The listing builds one solid part. Answer for the finished solid, in the listing's coordinates (mm). A direction names the side the tool comes from. Give positions to 0.01 mm unless a question says otherwise; leave off trailing zeros. Write each loop counter-clockwise with the first axis right and the second up, starting at its lowest first coordinate (ties: lowest second). Pieces come first, ordered by that corner, then holes. Notation, with made-up numbers: M -36.75,66 L 6.25,66 A33 ccw 6.25,105 Z; hole C -5.5,47 d5. An arc over 180 degrees is marked long. Return JSON: item names as keys, results as strings.
from build123d import *

# Parameters (mm, degrees)
SKETCH1_W           = 50.8
SKETCH1_H           = 50.8
SKETCH1_W_2         = 44.45
SKETCH1_H_2         = 44.45
BOSS_EXTRUDE1_DEPTH = 279.4
SKETCH2_R           = 6.35
SKETCH2_R_2         = 12.7
CUT_EXTRUDE1_DEPTH  = 289.488543967
CHAMFER1_SIZE       = 25.4
SKETCH3_R           = 3.175
CUT_EXTRUDE2_DEPTH  = 289.488543967
SKETCH4_W           = 25.4
SKETCH4_H           = 55.88
CUT_EXTRUDE3_DEPTH  = 289.488543967
CHAMFER2_SIZE       = 12.7
CUT_EXTRUDE5_REACH  = 290.489
SKETCH6_R           = 2.5796875


with BuildPart() as part:
    # Sketch1 → Boss-Extrude1 (new body)
    with BuildSketch(Plane(origin=(0, 0, 0), x_dir=(1, 0, 0), z_dir=(0, 1, 0))):
        with Locations((25.4, 25.4)):
            Rectangle(SKETCH1_W, SKETCH1_H)
        with Locations((25.4, 25.4)):
            Rectangle(SKETCH1_W_2, SKETCH1_H_2, mode=Mode.SUBTRACT)
    extrude(amount=BOSS_EXTRUDE1_DEPTH)

    # Sketch2 → Cut-Extrude1 (cut, through all)
    with BuildSketch(Plane(origin=(0, 0, -50.8), x_dir=(-1, 0, 0), z_dir=(0, 0, -1))):
        with Locations((-12.7, 25.4)):
            Circle(SKETCH2_R)
        with Locations((-25.4, 254)):
            Circle(SKETCH2_R_2)
    extrude(amount=-CUT_EXTRUDE1_DEPTH, mode=Mode.SUBTRACT)

    # Chamfer1
    # the kernel refuses this chamfer: 25.4 mm, written as the material it takes off along each edge
    with BuildSketch(Plane(origin=(50.8, 0, 65.320747894), x_dir=(-0.9996219169112966, -0.02749587661058637, 0), z_dir=(0, 0, -1))) as chamfer1_piece_1:
        Polygon((CHAMFER1_SIZE * 0.999621916911, CHAMFER1_SIZE * 0.0274958766106), (-CHAMFER1_SIZE * 0.0274958766106, CHAMFER1_SIZE * 0.999621916911), (0, 0), align=None)
    extrude(amount=181.441495789, mode=Mode.SUBTRACT)

    # Sketch3 → Cut-Extrude2 (cut, through all)
    with BuildSketch(Plane(origin=(0, 0, -50.8), x_dir=(-1, 0, 0), z_dir=(0, 0, -1))):
        with Locations((-38.1, 101.6)):
            Circle(SKETCH3_R)
    extrude(amount=-CUT_EXTRUDE2_DEPTH, mode=Mode.SUBTRACT)

    # Sketch4 → Cut-Extrude3 (cut, through all)
    with BuildSketch(Plane.ZY):
        with Locations((-38.1, 251.46)):
            Rectangle(SKETCH4_W, SKETCH4_H)
    extrude(amount=-CUT_EXTRUDE3_DEPTH, mode=Mode.SUBTRACT)

    # Chamfer2
    chamfer2_edges = [part.edges().sort_by_distance(p)[0] for p in [
        (49.2125, 279.4, -25.4),
        (1.5875, 279.4, -25.4),
    ]]
    chamfer(chamfer2_edges, length=CHAMFER2_SIZE)

    # Sketch6 → Cut-Extrude5 (cut, up to next)
    with BuildSketch(Plane.XY, mode=Mode.PRIVATE) as cut_extrude5_sk1:
        with Locations((7.439487758, 271.960512242)):
            Circle(SKETCH6_R)
    cut_extrude5_tool1 = extrude(cut_extrude5_sk1.sketch, amount=-CUT_EXTRUDE5_REACH, mode=Mode.PRIVATE) & part.part
    # Sketch6 → Cut-Extrude5 (cut, up to next)
    with BuildSketch(Plane.XY, mode=Mode.PRIVATE) as cut_extrude5_sk2:
        with Locations((7.439487758, 236.039487758)):
            Circle(SKETCH6_R)
    cut_extrude5_tool2 = extrude(cut_extrude5_sk2.sketch, amount=-CUT_EXTRUDE5_REACH, mode=Mode.PRIVATE) & part.part
    # Sketch6 → Cut-Extrude5 (cut, up to next)
    with BuildSketch(Plane.XY, mode=Mode.PRIVATE) as cut_extrude5_sk3:
        with Locations((43.360512242, 236.039487758)):
            Circle(SKETCH6_R)
    cut_extrude5_tool3 = extrude(cut_extrude5_sk3.sketch, amount=-CUT_EXTRUDE5_REACH, mode=Mode.PRIVATE) & part.part
    # Sketch6 → Cut-Extrude5 (cut, up to next)
    with BuildSketch(Plane.XY, mode=Mode.PRIVATE) as cut_extrude5_sk4:
        with Locations((43.360512242, 271.960512242)):
            Circle(SKETCH6_R)
    cut_extrude5_tool4 = extrude(cut_extrude5_sk4.sketch, amount=-CUT_EXTRUDE5_REACH, mode=Mode.PRIVATE) & part.part
    add(cut_extrude5_tool1.solids().sort_by_distance((7.439488, 271.960512, 0))[0], mode=Mode.SUBTRACT)
    add(cut_extrude5_tool2.solids().sort_by_distance((7.439488, 236.039488, 0))[0], mode=Mode.SUBTRACT)
    add(cut_extrude5_tool3.solids().sort_by_distance((43.360512, 236.039488, 0))[0], mode=Mode.SUBTRACT)
    add(cut_extrude5_tool4.solids().sort_by_distance((43.360512, 271.960512, 0))[0], mode=Mode.SUBTRACT)


solid = part.part
Item 1: Given pin 1 Ø6 at (x, y) = (43.36, 236.04) entering from -Z (3 decimals); pin 2 Ø3.5 at (x, y) = (2, 239.5) entering from -Z, each flat-ended and moving along its own axis, determine where each tip first touches the part or whether it passes through.
Geometry results:
{"pin 1": "stops at z = -3.175", "pin 2": "stops at z = -25.4"}
Item 2: A cutting plane is placed at C-C, the plane y = 101.6. Write down the section's boundary in (x, z) (3 decimals), plus the area to 3 significant figures.
Geometry results:
{"outline": "M 0,-50.8 L 34.925,-50.8 L 34.925,-47.625 L 3.175,-47.625 L 3.175,-3.175 L 34.925,-3.175 L 34.925,0 L 0,0 Z; M 41.275,-50.8 L 50.8,-50.8 L 50.8,0 L 41.275,0 L 41.275,-3.175 L 47.625,-3.175 L 47.625,-47.625 L 41.275,-47.625 Z", "area": "565 mm2"}
Item 3: A cutting plane is placed at D-D, the plane x = 16. Write down the section's boundary in (y, z) (3 decimals), plus the area to 3 significant figures.
Geometry results:
{"outline": "M 0,-50.8 L 19.975,-50.8 L 19.975,-47.625 L 0,-47.625 Z; M 0,-3.175 L 19.975,-3.175 L 19.975,0 L 0,0 Z; M 30.825,-50.8 L 223.52,-50.8 L 223.52,-47.625 L 30.825,-47.625 Z; M 30.825,-3.175 L 245.46,-3.175 L 245.46,0 L 30.825,0 Z; M 262.54,-3.175 L 279.4,-3.175 L 279.4,0 L 262.54,0 Z", "area": "1,470 mm2"}
Item 4: A cutting plane is placed at A-A, the plane z = -35.5. Write down the section's boundary in (x, y) (3 decimals).
Geometry results:
{"outline": "M 0,0 L 3.175,0 L 3.175,223.52 L 0,223.52 Z; M 47.625,22.225 L 50.8,25.4 L 50.8,223.52 L 47.625,223.52 Z"}
Item 5: Determine the mould class of faces 1 (the cylindrical face through (7.104, 238.597, -1.565)), 2 (the flat face through (48.4, 23, -23.4)), 3 (the flat face through (25, 110, -50.8)), 4 (the flat face through (0, 138, -25)) for opening direction X: +X half, -X half, draft (parallel to the pull), parting line (faces both ways), or undercut.
Geometry results:
{"face 1": "undercut", "face 2": "+X half", "face 3": "draft", "face 4": "-X half"}
Item 6: Which of the six approach directions +Z, -Z, +X, -X, +Y, -Y give full straight-line access (tool end or side, diameter ignored) to faces 5 (the cylindrical face through (40.44, 103.746, -1.61)), 6 (the flat face through (25, 223.52, -49)), 7 (the flat face through (47.625, 149, -25))?
Geometry results:
{"face 5": "+Z, -Z", "face 6": "-Z, +X, -X, +Y", "face 7": "+Y, -Y"}
Item 7: Find the intervals of material crossed by line 1 (Z direction, x = 33.5, y = 126) (3 decimals); line 2 (X direction, y = 113, z = -13) (3 decimals); line 3 (Y direction, x = 17.5, z = -3), in increasing order.
Geometry results:
{"line 1": "z = -50.8 to -47.625, -3.175 to 0", "line 2": "x = 0 to 3.175, 47.625 to 50.8", "line 3": "y = 0 to 21.24, 29.56 to 244.06, 263.94 to 279.4"}
Item 8: A cutting plane is placed at B-B, the plane y = 53. Write down the section's boundary in (x, z) (3 decimals).
Geometry results:
{"outline": "M 0,-50.8 L 50.8,-50.8 L 50.8,0 L 0,0 Z; hole M 3.175,-47.625 L 47.625,-47.625 L 47.625,-3.175 L 3.175,-3.175 Z"}
